```python
from build123d import *

# Parameters (mm, degrees)
CROQUIS1_R              = 1.628014373
SALIENTE_EXTRUIR1_DEPTH = 4
SALIENTE_EXTRUIR2_DEPTH = 9
CROQUIS3_R              = 1.5
CORTAR_EXTRUIR1_DEPTH   = 4
SALIENTE_EXTRUIR3_DEPTH = 7
CORTAR_EXTRUIR2_DEPTH   = 4.8
CROQUIS10_R             = 1
CORTAR_EXTRUIR3_DEPTH   = 4
SALIENTE_EXTRUIR4_START = 1
CROQUIS11_R             = 1
CROQUIS11_W             = 5.6
CROQUIS11_H             = 2.5
SALIENTE_EXTRUIR4_DEPTH = 1
CROQUIS12_W             = 27.503266124
CROQUIS12_H             = 20
CORTAR_EXTRUIR4_DEPTH   = 13
CROQUIS13_W             = 5.6
CROQUIS13_H             = 2.5
SALIENTE_EXTRUIR5_DEPTH = 1
SALIENTE_EXTRUIR6_DEPTH = 3
CROQUIS15_W             = 3
CROQUIS15_H             = 7
CORTAR_EXTRUIR5_DEPTH   = 3


with BuildPart() as part:
    # Croquis1 → Saliente-Extruir1 (new body)
    with BuildSketch(Plane.XY):
        with BuildLine():
            Line((-79.034482165, 42.285614206), (-79.034482165, 34.285614206))
            Line((-79.034482165, 34.285614206), (-85.534482165, 34.285614206))
            Line((-85.534482165, 34.285614206), (-85.534482165, 43.91362858))
            ThreePointArc((-85.534482165, 43.91362858), (-89.034482165, 47.41362858), (-92.534482165, 43.91362858))
            Line((-92.534482165, 43.91362858), (-92.534482165, 34.285614206))
            Line((-92.534482165, 34.285614206), (-99.034482165, 34.285614206))
            Line((-99.034482165, 34.285614206), (-99.034482165, 42.285614206))
            Line((-99.034482165, 42.285614206), (-99.034482165, 54.285614206))
            Line((-99.034482165, 54.285614206), (-79.034482165, 54.285614206))
            Line((-79.034482165, 54.285614206), (-79.034482165, 42.285614206))
        make_face()
        with Locations((-96.034482165, 38.285614206)):
            Circle(CROQUIS1_R, mode=Mode.SUBTRACT)
        with Locations((-82.034482165, 38.285614206)):
            Circle(CROQUIS1_R, mode=Mode.SUBTRACT)
    extrude(amount=SALIENTE_EXTRUIR1_DEPTH)

    # Croquis2 → Saliente-Extruir2 (add)
    with BuildSketch(Plane(origin=(0, 0, 0), x_dir=(-1, 0, 0), z_dir=(0, 0, -1))):
        with BuildLine():
            Line((79.034482165, 41.085614206), (83.629638531, 41.085614206))
            ThreePointArc((83.629638531, 41.085614206), (89.034482165, 50.01362858), (94.439325799, 41.085614206))
            Line((94.439325799, 41.085614206), (99.034482165, 41.085614206))
            Line((99.034482165, 41.085614206), (99.034482165, 54.285614206))
            Line((99.034482165, 54.285614206), (79.034482165, 54.285614206))
            Line((79.034482165, 54.285614206), (79.034482165, 41.085614206))
        make_face()
    extrude(amount=SALIENTE_EXTRUIR2_DEPTH)

    # Croquis3 → Cortar-Extruir1 (cut)
    with BuildSketch(Plane(origin=(0, 54.285614206, 0), x_dir=(1, 0, 0), z_dir=(0, 1, 0))):
        with Locations(Location((-90.034482165, 7, 0), (0, 0, 270))):
            Circle(CROQUIS3_R)
        with BuildLine():
            Line((-79.034482165, 8.118033989), (-79.034482165, 5.881966011))
            ThreePointArc((-79.034482165, 5.881966011), (-81.534482165, 7), (-79.034482165, 8.118033989))
        make_face()
    extrude(amount=-CORTAR_EXTRUIR1_DEPTH, mode=Mode.SUBTRACT)

    # Croquis4 → Saliente-Extruir3 (add)
    with BuildSketch(Plane(origin=(0, 54.285614206, 0), x_dir=(1, 0, 0), z_dir=(0, 1, 0))):
        with BuildLine():
            Line((-76.034482165, 1), (-76.034482165, 9))
            Line((-76.034482165, 9), (-79.034482165, 9))
            Line((-79.034482165, 9), (-79.034482165, 8.118033989))
            ThreePointArc((-79.034482165, 8.118033989), (-78.534482165, 7), (-79.034482165, 5.881966011))
            Line((-79.034482165, 5.881966011), (-79.034482165, -4))
            Line((-79.034482165, -4), (-76.034482165, 1))
        make_face()
    extrude(amount=-SALIENTE_EXTRUIR3_DEPTH)

    # Croquis5 → Cortar-Extruir2 (cut)
    with BuildSketch(Plane(origin=(0, 0, -9), x_dir=(-1, 0, 0), z_dir=(0, 0, -1))):
        Polygon((90.034482165, 50.285614206), (92.834482165, 50.285614206), (92.834482165, 52.785614206), (87.234482165, 52.785614206), (87.234482165, 50.285614206), align=None)
        Polygon((80.034482165, 50.285614206), (82.834482165, 50.285614206), (82.834482165, 52.785614206), (77.234482165, 52.785614206), (77.234482165, 50.285614206), align=None)
    extrude(amount=-CORTAR_EXTRUIR2_DEPTH, mode=Mode.SUBTRACT)

    # Croquis10 → Cortar-Extruir3 (cut)
    with BuildSketch(Plane(origin=(0, 0, -9), x_dir=(-1, 0, 0), z_dir=(0, 0, -1))):
        with Locations((96.534482165, 51.785614206)):
            Circle(CROQUIS10_R)
        with Locations((81.034482165, 43.085614206)):
            Circle(CROQUIS10_R)
    extrude(amount=-CORTAR_EXTRUIR3_DEPTH, mode=Mode.SUBTRACT)

    # Croquis11 → Saliente-Extruir4 (add)
    with BuildSketch(Plane(origin=(0, 0, -9), x_dir=(-1, 0, 0), z_dir=(0, 0, -1)).offset(SALIENTE_EXTRUIR4_START)):
        with BuildLine():
            Line((94.439325799, 41.085614206), (99.034482165, 41.085614206))
            Line((99.034482165, 41.085614206), (99.034482165, 54.285614206))
            Line((99.034482165, 54.285614206), (76.034482165, 54.285614206))
            Line((76.034482165, 54.285614206), (76.034482165, 47.285614206))
            Line((76.034482165, 47.285614206), (79.034482165, 47.285614206))
            Line((79.034482165, 47.285614206), (79.034482165, 41.085614206))
            Line((79.034482165, 41.085614206), (83.629638531, 41.085614206))
            Line((83.629638531, 41.085614206), (84.911093424, 41.085614206))
            ThreePointArc((84.911093424, 41.085614206), (89.034482165, 48.91362858), (93.157870905, 41.085614206))
            Line((93.157870905, 41.085614206), (94.439325799, 41.085614206))
        make_face()
        with Locations((96.534482165, 51.785614206)):
            Circle(CROQUIS11_R, mode=Mode.SUBTRACT)
        with Locations((81.034482165, 43.085614206)):
            Circle(CROQUIS11_R, mode=Mode.SUBTRACT)
        with Locations((90.034482165, 51.535614206)):
            Rectangle(CROQUIS11_W, CROQUIS11_H, mode=Mode.SUBTRACT)
        with Locations((80.034482165, 51.535614206)):
            Rectangle(CROQUIS11_W, CROQUIS11_H, mode=Mode.SUBTRACT)
    extrude(amount=-SALIENTE_EXTRUIR4_DEPTH)

    # Croquis12 → Cortar-Extruir4 (cut)
    with BuildSketch(Plane.XY.offset(4)):
        with Locations((-85.282849103, 44.285614206)):
            Rectangle(CROQUIS12_W, CROQUIS12_H)
    extrude(amount=-CORTAR_EXTRUIR4_DEPTH, mode=Mode.SUBTRACT)

    # Croquis13 → Saliente-Extruir5 (add)
    with BuildSketch(Plane(origin=(0, 0, -10), x_dir=(-1, 0, 0), z_dir=(0, 0, -1))):
        with Locations((90.034482165, 51.535614206)):
            Rectangle(CROQUIS13_W, CROQUIS13_H)
        with Locations((80.034482165, 51.535614206)):
            Rectangle(CROQUIS13_W, CROQUIS13_H)
    extrude(amount=-SALIENTE_EXTRUIR5_DEPTH)

    # Croquis14 → Saliente-Extruir6 (add)
    with BuildSketch(Plane(origin=(0, 0, -10), x_dir=(-1, 0, 0), z_dir=(0, 0, -1))):
        with BuildLine():
            Line((99.034482165, 41.085614206), (99.034482165, 38.085614206))
            Line((99.034482165, 38.085614206), (79.034482165, 38.085614206))
            Line((79.034482165, 38.085614206), (79.034482165, 41.085614206))
            Line((79.034482165, 41.085614206), (84.911093424, 41.085614206))
            ThreePointArc((84.911093424, 41.085614206), (89.034482165, 39.377650667), (93.157870905, 41.085614206))
            Line((93.157870905, 41.085614206), (99.034482165, 41.085614206))
        make_face()
    extrude(amount=-SALIENTE_EXTRUIR6_DEPTH)

    # Croquis15 → Cortar-Extruir5 (cut)
    with BuildSketch(Plane(origin=(0, 0, -10), x_dir=(-1, 0, 0), z_dir=(0, 0, -1))):
        with Locations((77.534482165, 50.785614206)):
            Rectangle(CROQUIS15_W, CROQUIS15_H)
    extrude(amount=-CORTAR_EXTRUIR5_DEPTH, mode=Mode.SUBTRACT)


solid = part.part
```
Input: part model. Units: mm. Frame: model coordinates. A direction names the side the tool comes from. Give positions to 0.01 mm unless a question says otherwise; leave off trailing zeros. Loops run counter-clockwise (first coordinate to the right, second up) from the corner with the lowest first, then second, coordinate; pieces in that order, holes last.
1) Section query C-C on y = 42.5. Return the cut outline in (x, z).
A:
outline: (-99.03, -10) - (-93.83, -10) - (-93.83, -9) - (-99.03, -9) - close; (-84.24, -10) - (-81.85, -10) - (-81.85, -9) - (-84.24, -9) - close; (-80.22, -10) - (-79.03, -10) - (-79.03, -9) - (-80.22, -9) - close
2) Contact query for flat-ended pins moving along their axis: pin 1 (8 mm diameter, centred on x = -86.5, y = 40, fed in from -Z); pin 2 (0.6 mm diameter, centred on x = -82, z = -8, fed in from +Y); pin 3 (1.8 mm diameter, centred on x = -81.03, y = 43.09, fed in from +Z); pin 4 (3 mm diameter, centred on x = -96.53, y = 51.79, fed in from +Z). Output: stop coordinate, or through.
A:
pin 1: stops at z = -10
pin 2: stops at y = 41.09
pin 3: passes through
pin 4: stops at z = -9
3) Line query: L1, parallel to X at y = 43, z = -9.6; L2, parallel to Z at x = -83.25, y = 49.25; L3, parallel to Y at x = -96, z = -7.6. Output: solid intervals per line, ascending.
A:
L1: x = -99.03 to -93.95, -84.12 to -82.03, -80.04 to -79.03
L2: z = -10 to -9
L3: y = 38.09 to 41.09
4) Section query D-D on z = -7.7. Return the cut outline in (x, y).
A:
outline: (-99.03, 38.09) - (-79.03, 38.09) - (-79.03, 41.09) - (-84.91, 41.09) arc R5.83 cw to (-93.16, 41.09) - (-99.03, 41.09) - close
5) Section query B-B on y = 46. Return the cut outline in (x, z), and give its area (3 significant figures).
A:
outline: (-99.03, -10) - (-93.58, -10) - (-93.58, -9) - (-99.03, -9) - close; (-84.49, -10) - (-79.03, -10) - (-79.03, -9) - (-84.49, -9) - close
area: 10.9 mm2
6) Section query A-A on x = -87. Return the cut outline in (y, z), and give its area (3 significant figures).
A:
outline: (38.09, -10) - (39.74, -10) - (39.74, -7) - (38.09, -7) - close; (48.48, -10) - (54.29, -10) - (54.29, -9) - (48.48, -9) - close
area: 10.8 mm2
7) Reachability of faces 4 (the flat face through (-89, 38.086, -9)), 5 (the flat face through (-89.2, 49.2, -9)), 6 (the cylindrical face through (-88.97, 39.38, -8.52)) from +Z, -Z, +X, -X, +Y, -Y: full face, straight path, thin tool, end or side. Return the list, or none.
A:
face 4: +Z, -Z, +X, -X, -Y
face 5: +Z, +X, -X, +Y
face 6: +Z, -Z
8) Mould query, pull axis X, two halves, no side actions, for faces 1 (the flat face through (-89, 39, -7)), 2 (the flat face through (-79.034, 44.3, -9.2)), 3 (the cylindrical face through (-97.07, 52.63, -9.51)). Classes: released by +X, released by -X, zero draft, split by the parting line, or undercut.
A:
face 1: zero draft
face 2: released by +X
face 3: undercut
